Geometry check sheet. Reference: drawing and pictorial views, mm from the part's lowest x, y, z. A direction names the side the tool comes from. Coordinates: 2 decimals unless noted, no trailing zeros. Loops run counter-clockwise (first coordinate to the right, second up) from the corner with the lowest first, then second, coordinate; pieces in that order, holes last. Notation, with made-up numbers: (22, 74.25) - (76, 74.25) arc R9 cw to (76, 87.25) - close; hole circle Ø1 at (37.25, 16.5). An arc over 180 degrees is marked (long way). One line per item, written item: value.
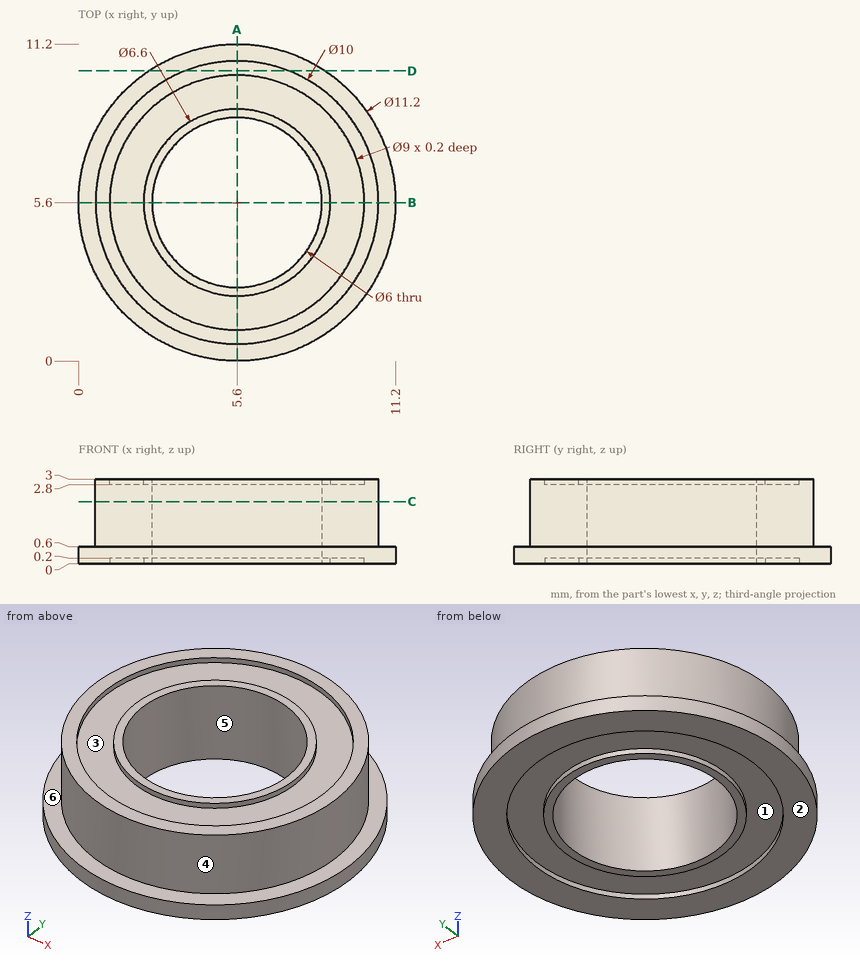
(1) Material ranges on probe 1 along Y at (x, z) = (5.6, 2.95); probe 2 along Y at (x, z) = (5.6, 1.15); probe 3 along Y at (x, z) = (5.6, 0.1), recorded low to high. Write a range as from..to.
Reply:
probe 1: 0.6..1.1, 2.3..2.6, 8.6..8.9, 10.1..10.6
probe 2: 0.6..2.6, 8.6..10.6
probe 3: 0..1.1, 2.3..2.6, 8.6..8.9, 10.1..11.2
(2) Cross-section at A-A on x = 5.6. Record the cut outline in (y, z), and give its area (3 significant figures).
Reply:
outline: (0, 0) - (1.1, 0) - (1.1, 0.2) - (2.3, 0.2) - (2.3, 0) - (2.6, 0) - (2.6, 3) - (2.3, 3) - (2.3, 2.8) - (1.1, 2.8) - (1.1, 3) - (0.6, 3) - (0.6, 0.6) - (0, 0.6) - close; (8.6, 0) - (8.9, 0) - (8.9, 0.2) - (10.1, 0.2) - (10.1, 0) - (11.2, 0) - (11.2, 0.6) - (10.6, 0.6) - (10.6, 3) - (10.1, 3) - (10.1, 2.8) - (8.9, 2.8) - (8.9, 3) - (8.6, 3) - close
area: 11.8 mm2
(3) Access from +Z, -Z, +X, -X, +Y, -Y to the whole of each face (thin tool, end or side, straight path). Record for the marked faces 5 and 6.
Reply:
face 5: +Z, -Z
face 6: +Z
(4) Cross-section at C-C on z = 2.2. Record the cut outline in (x, y).
Reply:
outline: circle Ø10 at (5.6, 5.6); hole circle Ø6 at (5.6, 5.6)
(5) Go/stop test with flat-tipped pins: pin 1 Ø1 at (y, z) = (9.5, 2.5) entering from -X; pin 2 Ø1.5 at (x, z) = (3.5, 1) entering from +Y; pin 3 Ø1 at (y, z) = (5, 1.5) entering from -X. Record where each tip stops, or that it passes through.
Reply:
pin 1: x = 1.93
pin 2: y = 11
pin 3: x = 0.6
(6) Release check for a two-part mould opening along Y. For the marked faces 1, 2, 3 and 4 record: pulls with the +Y half, pulls with the -Y half, needs draft (parallel to the pull), parting line crosses it, or undercut.
Reply:
face 1: undercut
face 2: needs draft
face 3: undercut
face 4: parting line crosses it
(7) Cross-section at D-D on y = 10.25. Record the cut outline in (x, z).
Reply:
outline: (2.48, 0) - (8.72, 0) - (8.72, 0.6) - (7.44, 0.6) - (7.44, 3) - (3.76, 3) - (3.76, 0.6) - (2.48, 0.6) - close
